from build123d import *

# Parameters (mm, degrees)
SKETCH_1_W          = 42
SKETCH_1_H          = 42
EXTRUDE_1_DEPTH     = 1.6
SKETCH_2_R          = 1.5
CUT_EXTRUDE_1_DEPTH = 2.6
SKETCH_3_R          = 3.4
EXTRUDE_2_DEPTH     = 1.2
SKETCH_4_R          = 1.5
CUT_EXTRUDE_2_DEPTH = 10


with BuildPart() as part:
    # 草图1 → 凸台-拉伸1 (new body)
    with BuildSketch(Plane(origin=(0, 0, 0), x_dir=(1, 0, 0), z_dir=(0, 1, 0))):
        with Locations((21, 21)):
            Rectangle(SKETCH_1_W, SKETCH_1_H)
    extrude(amount=EXTRUDE_1_DEPTH)

    # 草图2 → 切除-拉伸1 (cut, through all)
    with BuildSketch(Plane(origin=(0, 1.6, 0), x_dir=(1, 0, 0), z_dir=(0, 1, 0))):
        with Locations((5.5, 36.5)):
            Circle(SKETCH_2_R)
        with Locations((36.5, 36.5)):
            Circle(SKETCH_2_R)
        with Locations((5.5, 5.5)):
            Circle(SKETCH_2_R)
        with Locations((36.5, 5.5)):
            Circle(SKETCH_2_R)
    extrude(amount=-CUT_EXTRUDE_1_DEPTH, mode=Mode.SUBTRACT)

    # 草图3 → 凸台-拉伸2 (add)
    with BuildSketch(Plane(origin=(0, 1.6, 0), x_dir=(1, 0, 0), z_dir=(0, 1, 0))):
        with Locations((21, 21)):
            Circle(SKETCH_3_R)
    extrude(amount=EXTRUDE_2_DEPTH)

    # 草图4 → 切除-拉伸2 (cut)
    with BuildSketch(Plane(origin=(0, 1.6, 0), x_dir=(1, 0, 0), z_dir=(0, 1, 0))):
        with Locations((14.282485579, 27.717514421)):
            Circle(SKETCH_4_R)
        with Locations((27.717514421, 27.717514421)):
            Circle(SKETCH_4_R)
        with Locations((14.282485579, 14.282485579)):
            Circle(SKETCH_4_R)
        with Locations((27.717514421, 14.282485579)):
            Circle(SKETCH_4_R)
    extrude(amount=-CUT_EXTRUDE_2_DEPTH, mode=Mode.SUBTRACT)


solid = part.part
Geometry check sheet. Reference: the model listing, model coordinates, mm. Coordinates: 2 decimals unless noted, no trailing zeros. Order: outer loops, then holes, each group sorted by start corner. A loop starts at its lowest first (then second) coordinate and runs counter-clockwise, first axis right, second up. Notation, with made-up numbers: (70.25, -2) -> (121.25, -2) arc R31 cw to (121.25, 33) -> close; hole circle Ø8 at (-6.75, 38). An arc over 180 degrees is marked (long way). Use a Markdown table: item, result. Add a question column.
1. Cross-section at A-A (z = -5.5). Enter the section's corners in (x, y), and give its area (3 significant figures).
2. Cross-section at D-D (x = 21). Enter the section's corners in (y, z).
3. Cross-section at C-C (z = -21). Enter the section's corners in (x, y), and give its area (3 significant figures).
4. Mould release check, pull along Z, two halves, no side actions. Record for faces 1 (the face through (24.243, 2.192, -22.021)), 2 (the face through (42, 1, -21)), 3 (the face through (4.3, 0.8, -4.6)): pulls with the +Z half, pulls with the -Z half, needs draft (parallel to the pull), parting line crosses it, or undercut.
5. Material ranges on L1, parallel to X at y = 0.9, z = -5.5; L2, parallel to Z at x = 36.5, y = 1.1; L3, parallel to Y at x = 33.5, z = -21.5, recorded low to high.
6. Go/stop test with flat-tipped pins: pin 1 Ø1 at (x, y) = (18.5, 2.5) entering from -Z; pin 2 Ø2 at (x, z) = (13, -26) entering from +Y. Record where each tip stops, or that it passes through.
7. Cross-section at B-B (x = 36.5). Enter the section's corners in (y, z).
Filled sheet:
| question | item | result |
|---|---|---|
| 1 | outline | (0, 0) -> (4, 0) -> (4, 1.6) -> (0, 1.6) -> close; (7, 0) -> (35, 0) -> (35, 1.6) -> (7, 1.6) -> close; (38, 0) -> (42, 0) -> (42, 1.6) -> (38, 1.6) -> close |
| 1 | area | 57.6 mm2 |
| 2 | outline | (0, -42) -> (1.6, -42) -> (1.6, -24.4) -> (2.8, -24.4) -> (2.8, -17.6) -> (1.6, -17.6) -> (1.6, 0) -> (0, 0) -> close |
| 3 | outline | (0, 0) -> (42, 0) -> (42, 1.6) -> (24.4, 1.6) -> (24.4, 2.8) -> (17.6, 2.8) -> (17.6, 1.6) -> (0, 1.6) -> close |
| 3 | area | 75.4 mm2 |
| 4 | face 1 | parting line crosses it |
| 4 | face 2 | needs draft |
| 4 | face 3 | undercut |
| 5 | L1 | 0 to 4, 7 to 35, 38 to 42 |
| 5 | L2 | -42 to -38, -35 to -7, -4 to 0 |
| 5 | L3 | 0 to 1.6 |
| 6 | pin 1 | z = -23.75 |
| 6 | pin 2 | y = 1.6 |
| 7 | outline | (0, -42) -> (1.6, -42) -> (1.6, -38) -> (0, -38) -> close; (0, -35) -> (1.6, -35) -> (1.6, -7) -> (0, -7) -> close; (0, -4) -> (1.6, -4) -> (1.6, 0) -> (0, 0) -> close |
